Part model, mm, in its own coordinate system. Give positions to 0.01 mm unless a question says otherwise; leave off trailing zeros. Write each loop counter-clockwise with the first axis right and the second up, starting at its lowest first coordinate (ties: lowest second). Pieces come first, ordered by that corner, then holes. Notation, with made-up numbers: (33, -36.5) - (92, -36.5) arc R18 ccw to (92, -20.5) - close; hole circle Ø6 at (40.25, 21.25). An arc over 180 degrees is marked (long way). Answer as a JSON object with one key per item and string values. Group by question number.
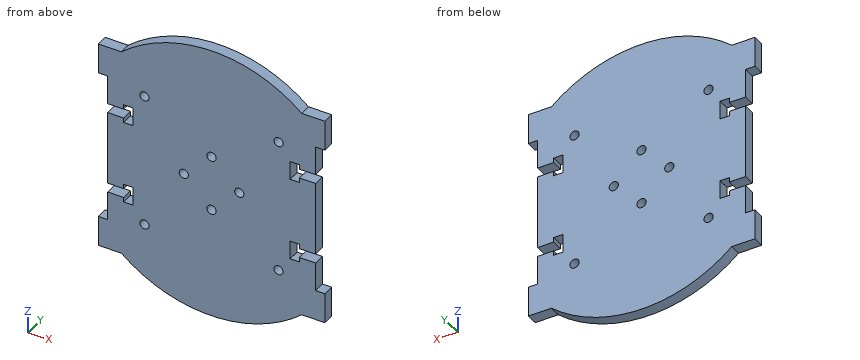
```python
from build123d import *

# Parameters (mm, degrees)
SKETCH1_R           = 2
BOSS_EXTRUDE1_DEPTH = 5


with BuildPart() as part:
    # Sketch1 → Boss-Extrude1 (new body)
    with BuildSketch(Plane(origin=(0, 0, 0), x_dir=(1, 0, 0), z_dir=(0, 1, 0))):
        with BuildLine():
            Line((-49, 45.6), (-49, 32.5))
            Line((-49, 32.5), (-45, 32.5))
            Line((-45, 32.5), (-45, 20))
            Line((-45, 20), (-38, 20))
            Line((-38, 20), (-38, 22))
            Line((-38, 22), (-34, 22))
            Line((-34, 22), (-34, 14))
            Line((-34, 14), (-38, 14))
            Line((-38, 14), (-38, 16))
            Line((-38, 16), (-45, 16))
            Line((-45, 16), (-45, -16))
            Line((-45, -16), (-38, -16))
            Line((-38, -16), (-38, -14))
            Line((-38, -14), (-34, -14))
            Line((-34, -14), (-34, -22))
            Line((-34, -22), (-38, -22))
            Line((-38, -22), (-38, -20))
            Line((-38, -20), (-45, -20))
            Line((-45, -20), (-45, -32.5))
            Line((-45, -32.5), (-49, -32.5))
            Line((-49, -32.5), (-49, -45.6))
            Line((-49, -45.6), (-39, -45.6))
            ThreePointArc((-39, -45.6), (0, -60.002999925), (39, -45.6))
            Line((39, -45.6), (49, -45.6))
            Line((49, -45.6), (49, -32.5))
            Line((49, -32.5), (45, -32.5))
            Line((45, -32.5), (45, -20))
            Line((45, -20), (38, -20))
            Line((38, -20), (38, -22))
            Line((38, -22), (34, -22))
            Line((34, -22), (34, -14))
            Line((34, -14), (38, -14))
            Line((38, -14), (38, -16))
            Line((38, -16), (45, -16))
            Line((45, -16), (45, 16))
            Line((45, 16), (38, 16))
            Line((38, 16), (38, 14))
            Line((38, 14), (34, 14))
            Line((34, 14), (34, 22))
            Line((34, 22), (38, 22))
            Line((38, 22), (38, 20))
            Line((38, 20), (45, 20))
            Line((45, 20), (45, 32.5))
            Line((45, 32.5), (49, 32.5))
            Line((49, 32.5), (49, 45.6))
            Line((49, 45.6), (38.995384342, 45.6))
            ThreePointArc((38.995384342, 45.6), (0, 60), (-38.995384342, 45.6))
            Line((-38.995384342, 45.6), (-49, 45.6))
        make_face()
        with Locations((-12, 0)):
            Circle(SKETCH1_R, mode=Mode.SUBTRACT)
        with Locations((0, 12)):
            Circle(SKETCH1_R, mode=Mode.SUBTRACT)
        with Locations((12, 0)):
            Circle(SKETCH1_R, mode=Mode.SUBTRACT)
        with Locations((0, -12)):
            Circle(SKETCH1_R, mode=Mode.SUBTRACT)
        with Locations((29, 29)):
            Circle(SKETCH1_R, mode=Mode.SUBTRACT)
        with Locations((29, -29)):
            Circle(SKETCH1_R, mode=Mode.SUBTRACT)
        with Locations((-29, -29)):
            Circle(SKETCH1_R, mode=Mode.SUBTRACT)
        with Locations((-29, 29)):
            Circle(SKETCH1_R, mode=Mode.SUBTRACT)
    extrude(amount=BOSS_EXTRUDE1_DEPTH)


solid = part.part
```
1) Band-saw the part on B-B (x = 0). List the corners of the cut face in (y, z).
2) Probe line 1 (Z direction, x = -44.5, y = 0.3); line 2 (X direction, y = 2.05, z = -29); line 3 (Z direction, x = -29, y = 2.4). List the from-to ranges inside material, lowest first.
3) Band-saw the part on A-A (z = 12). List the corners of the cut face in (x, y).
4) Band-saw the part on C-C (x = 12). List the corners of the cut face in (y, z).
5) Drop flat-ended pins along their axis: P1, Ø1.5, axis at y = 3, z = -29, coming from the -X side; P2, Ø3.5, axis at x = 0, z = -12, coming from the +Y side; P3, Ø1.5, axis at x = -40.5, y = 2, coming from the -Z side; P4, Ø3, axis at x = 35.5, y = 2, coming from the +Z side. Give the stop position or say it passes through.
6) Band-saw the part on D-D (y = 1.55). State how many separate pieces and enclosed holes the cut face has, plus the area to 3 significant figures.
Verdict:
{
 "1": {"outline": "(0, -60) - (5, -60) - (5, -14) - (0, -14) - close; (0, -10) - (5, -10) - (5, 10) - (0, 10) - close; (0, 14) - (5, 14) - (5, 60) - (0, 60) - close"},
 "2": {"line 1": "-45.6 to -20, -16 to 16, 20 to 45.6", "line 2": "-45 to -31, -27 to 27, 31 to 45", "line 3": "-52.53 to -31, -27 to 27, 31 to 52.53"},
 "3": {"outline": "(-45, 0) - (-2, 0) - (-2, 5) - (-45, 5) - close; (2, 0) - (45, 0) - (45, 5) - (2, 5) - close"},
 "4": {"outline": "(0, -58.79) - (5, -58.79) - (5, -2) - (0, -2) - close; (0, 2) - (5, 2) - (5, 58.79) - (0, 58.79) - close"},
 "5": {"P1": "x = -45", "P2": "through", "P3": "z = -45.6", "P4": "z = 49.44"},
 "6": {"separate pieces": "1", "enclosed holes": "8", "area": "9,610 mm2"}
}
